from build123d import *

# Parameters (mm, degrees)
SKETCH_W        = 1028.7
SKETCH_H        = 762
PAD_DEPTH       = 2133.6
SKETCH001_W     = 825.5
SKETCH001_H     = 406.4
POCKET_DEPTH    = 2133.601
SKETCH002_W     = 507.999996
SKETCH002_H     = 2032
POCKET001_DEPTH = 1028.701
SKETCH003_W     = 101.600004
SKETCH003_H     = 2032
POCKET002_DEPTH = 1028.701


with BuildPart() as part:
    # Sketch → Pad (new body)
    with BuildSketch(Plane.XZ):
        Rectangle(SKETCH_W, SKETCH_H)
    extrude(amount=PAD_DEPTH)

    # Sketch001 → Pocket (cut, through all)
    with BuildSketch(Plane(origin=(0, -2133.6, 0), x_dir=(1, 0, 0), z_dir=(0, -1, 0))):
        with Locations((0, -76.2)):
            Rectangle(SKETCH001_W, SKETCH001_H)
    extrude(amount=-POCKET_DEPTH, mode=Mode.SUBTRACT)

    # Sketch002 → Pocket001 (cut, through all)
    with BuildSketch(Plane(origin=(514.35, 0, 0), x_dir=(0, 0, 1), z_dir=(1, 0, 0))):
        with Locations((-127.000002, 1066.8)):
            Rectangle(SKETCH002_W, SKETCH002_H)
    extrude(amount=-POCKET001_DEPTH, mode=Mode.SUBTRACT)

    # Sketch003 → Pocket002 (cut, through all)
    with BuildSketch(Plane(origin=(514.35, 0, 0), x_dir=(0, 0, 1), z_dir=(1, 0, 0))):
        with Locations((330.199998, 1066.8)):
            Rectangle(SKETCH003_W, SKETCH003_H)
    extrude(amount=-POCKET002_DEPTH, mode=Mode.SUBTRACT)


solid = part.part
The model under review builds one solid part; all positions refer to its coordinate system, in mm. A direction names the side the tool comes from. Round coordinates to 2 decimals unless told otherwise and drop trailing zeros. Order: outer loops, then holes, each group sorted by start corner. A loop starts at its lowest first (then second) coordinate and runs counter-clockwise, first axis right, second up. Notation, with made-up numbers: (16, -29) -> (52, -29) arc R31 ccw to (52, -1) -> close; hole circle Ø2 at (81, 4). An arc over 180 degrees is marked (long way). Use CSV: the item, a comma, the result in double quotes. Start each with the question number.
(1) Tool access review of faces 5 (the face through (7, -50.8, -300)), 6 (the face through (412.75, -44, -77)), 7 (the face through (-7, -25, 381)), 8 (the face through (-7, -25, -381)), 9 (the face through (7, -50.8, 329)): name each direction out of +Z, -Z, +X, -X, +Y, -Y from which nothing blocks a thin tool from reaching the whole face with its end or side.
(2) Wall thickness on probe 1 along Y at (x, z) = (257.5, -347.5); probe 2 along Z at (x, y) = (-445, -1259.5): over which ranges is each line inside the solid? List them lowest first. Write a range as from..to.
(3) Consider section A-A on z = -202. Write out the cut boundary in (x, y).
(4) Mouldability with a two-part tool opening along X and no side actions: class faces 1 (the face through (514.35, -1220, 168)), 2 (the face through (-412.75, -44, -77)), 3 (the face through (-6, -2109, -279.4)), 4 (the face through (464, -1053, 127)) as pulls with the +X half, pulls with the -X half, needs draft (parallel to the pull), parting line crosses it, or undercut.
(5) Consider section B-B on x = 148. Write out the cut boundary in (y, z), and give its area (3 significant figures).
(6) Insertion check: pin 1 (8 mm diameter, centred on x = 25, y = -1467, fed in from -Z); pin 2 (2 mm diameter, centred on x = -208, y = -1762.5, fed in from +Z). Each pin has a flat end and moves straight along its axis. Give the tip position at first contact, or say it passes through.
Responses:
1,face 5,"-Z, +X, -X"
1,face 6,"+Y, -Y"
1,face 7,"+Z, +X, -X, +Y, -Y"
1,face 8,"-Z, +X, -X, +Y, -Y"
1,face 9,"+Z, +X, -X"
2,probe 1,"-2133.6..-2082.8, -50.8..0"
2,probe 2,"127..279.4"
3,outline,"(-514.35, -2133.6) -> (-412.75, -2133.6) -> (-412.75, -2082.8) -> (-514.35, -2082.8) -> close; (-514.35, -50.8) -> (-412.75, -50.8) -> (-412.75, 0) -> (-514.35, 0) -> close; (412.75, -2133.6) -> (514.35, -2133.6) -> (514.35, -2082.8) -> (412.75, -2082.8) -> close; (412.75, -50.8) -> (514.35, -50.8) -> (514.35, 0) -> (412.75, 0) -> close"
4,face 1,"pulls with the +X half"
4,face 2,"undercut"
4,face 3,"undercut"
4,face 4,"needs draft"
5,outline,"(-2133.6, -381) -> (-2082.8, -381) -> (-2082.8, -279.4) -> (-2133.6, -279.4) -> close; (-2133.6, 127) -> (0, 127) -> (0, 381) -> (-50.8, 381) -> (-50.8, 279.4) -> (-2082.8, 279.4) -> (-2082.8, 381) -> (-2133.6, 381) -> close; (-50.8, -381) -> (0, -381) -> (0, -279.4) -> (-50.8, -279.4) -> close"
5,area,"346,000 mm²"
6,pin 1,"z = 127"
6,pin 2,"z = 279.4"
